from build123d import *

# Parameters (mm, degrees)
SKETCH1_R           = 1.5
BOSS_EXTRUDE1_DEPTH = 3
FILLET1_R           = 1


with BuildPart() as part:
    # Sketch1 → Boss-Extrude1 (new body)
    with BuildSketch(Plane.XY):
        with BuildLine():
            Line((-2.5, 0), (-2.5, -37.136851725))
            Line((-2.5, -37.136851725), (-7.28143986, -46.828388088))
            ThreePointArc((-7.28143986, -46.828388088), (-6.145564068, -50.176489966), (-2.79746219, -49.040614175))
            Line((-2.79746219, -49.040614175), (2.5, -38.303148275))
            Line((2.5, -38.303148275), (2.5, 0))
            ThreePointArc((2.5, 0), (0, 2.5), (-2.5, 0))
        make_face()
        Circle(SKETCH1_R, mode=Mode.SUBTRACT)
        with Locations((-5.039451025, -47.934501132)):
            Circle(SKETCH1_R, mode=Mode.SUBTRACT)
    extrude(amount=BOSS_EXTRUDE1_DEPTH)

    # Fillet1
    # the kernel refuses this fillet: 1 mm, written as the material it adds along each edge
    with BuildSketch(Plane(origin=(-2.5, -37.136851725, 0), x_dir=(0, 1, 0), z_dir=(0, 0, 1))) as fillet1_piece_1:
        with BuildLine():
            CenterArc((FILLET1_R * 0.23325930992, FILLET1_R), FILLET1_R, 243.74, 26.26)
            Line((-FILLET1_R * 0.209185907385, FILLET1_R * 0.103204466066), (0, 0))
            Line((0, 0), (FILLET1_R * 0.23325930992, 0))
        make_face()
    extrude(amount=3)
    # the kernel refuses this fillet: 1 mm, written as the material it takes off along each edge
    with BuildSketch(Plane(origin=(1.5, -38.069888965, 2), x_dir=(0.8967955339340403, -0.44244521730487674, 0), z_dir=(0, 0, 1))) as fillet1_2_piece_1_section:
        Polygon((0, 0), (FILLET1_R, 0), (FILLET1_R, FILLET1_R * 0.23325930992), (FILLET1_R * 0.896795533934, FILLET1_R * 0.442445217305), align=None)
    fillet1_2_piece_1 = extrude(amount=FILLET1_R, mode=Mode.PRIVATE)
    fillet1_2_piece_1 = fillet1_2_piece_1 - Plane(origin=(1.5, -38.069888965, 2), x_dir=(-0.9738571594268947, 0.22716124896861223, 0), z_dir=(0, 0, 1)) * Sphere(FILLET1_R, mode=Mode.PRIVATE)
    add(fillet1_2_piece_1, mode=Mode.SUBTRACT)
    with BuildSketch(Plane(origin=(1.5, -38.069888965, 1), x_dir=(0.8967955339340403, -0.44244521730487674, 0), z_dir=(0, 0, -1))) as fillet1_2_piece_2_section:
        Polygon((0, 0), (FILLET1_R, 0), (FILLET1_R, -FILLET1_R * 0.23325930992), (FILLET1_R * 0.896795533934, -FILLET1_R * 0.442445217305), align=None)
    fillet1_2_piece_2 = extrude(amount=FILLET1_R, mode=Mode.PRIVATE)
    fillet1_2_piece_2 = fillet1_2_piece_2 - Plane(origin=(1.5, -38.069888965, 1), x_dir=(-0.9738571594268947, 0.22716124896861223, 0), z_dir=(0, 0, -1)) * Sphere(FILLET1_R, mode=Mode.PRIVATE)
    add(fillet1_2_piece_2, mode=Mode.SUBTRACT)
    with BuildSketch(Plane(origin=(0, 0, 3), x_dir=(1, 0, 0), z_dir=(0, -1, 0))) as fillet1_2_piece_3:
        with BuildLine():
            CenterArc((2.5 - FILLET1_R, -FILLET1_R), FILLET1_R, 0, 90)
            Line((2.5, -FILLET1_R), (2.5, 0))
            Line((2.5, 0), (2.5 - FILLET1_R, 0))
        make_face()
    revolve(axis=Axis((0, 0, 3), (0, 0, 1)), revolution_arc=180, mode=Mode.SUBTRACT)
    with BuildSketch(Plane(origin=(0, 0, 0), x_dir=(1, 0, 0), z_dir=(0, -1, 0))) as fillet1_2_piece_4:
        with BuildLine():
            CenterArc((2.5 - FILLET1_R, FILLET1_R), FILLET1_R, 270, 90)
            Line((2.5, FILLET1_R), (2.5, 0))
            Line((2.5, 0), (2.5 - FILLET1_R, 0))
        make_face()
    revolve(axis=Axis((0, 0, 0), (0, 0, 1)), revolution_arc=180, mode=Mode.SUBTRACT)
    with BuildSketch(Plane(origin=(-2.5, 0, 3), x_dir=(0, 0, -1), z_dir=(0, -1, 0))) as fillet1_2_piece_5:
        with BuildLine():
            CenterArc((FILLET1_R, FILLET1_R), FILLET1_R, 180, 90)
            Line((0, FILLET1_R), (0, 0))
            Line((0, 0), (FILLET1_R, 0))
        make_face()
    extrude(amount=36.903592415, mode=Mode.SUBTRACT)
    with BuildSketch(Plane(origin=(-2.5, 0, 0), x_dir=(0, 0, 1), z_dir=(0, -1, 0))) as fillet1_2_piece_6:
        with BuildLine():
            CenterArc((FILLET1_R, -FILLET1_R), FILLET1_R, 90, 90)
            Line((0, -FILLET1_R), (0, 0))
            Line((0, 0), (FILLET1_R, 0))
        make_face()
    extrude(amount=36.903592415, mode=Mode.SUBTRACT)
    with BuildSketch(Plane(origin=(-2.603204466, -37.346037633, 3), x_dir=(0.8967955339340403, -0.4424452173048767, 0), z_dir=(-0.4424452173048767, -0.8967955339340403, 0))) as fillet1_2_piece_7:
        with BuildLine():
            CenterArc((FILLET1_R, -FILLET1_R), FILLET1_R, 90, 90)
            Line((0, -FILLET1_R), (0, 0))
            Line((0, 0), (FILLET1_R, 0))
        make_face()
    extrude(amount=10.573592415, mode=Mode.SUBTRACT)
    with BuildSketch(Plane(origin=(-2.603204466, -37.346037633, 0), x_dir=(0.8967955339340403, -0.4424452173048767, 0), z_dir=(-0.4424452173048767, -0.8967955339340403, 0))) as fillet1_2_piece_8:
        with BuildLine():
            CenterArc((FILLET1_R, FILLET1_R), FILLET1_R, 180, 90)
            Line((0, FILLET1_R), (0, 0))
            Line((0, 0), (FILLET1_R, 0))
        make_face()
    extrude(amount=10.573592415, mode=Mode.SUBTRACT)
    with BuildSketch(Plane(origin=(-5.039451025, -47.934501132, 3), x_dir=(-0.8967955339340404, 0.44244521730487624, 0), z_dir=(0.44244521730487624, 0.8967955339340404, 0))) as fillet1_2_piece_9:
        with BuildLine():
            CenterArc((2.5 - FILLET1_R, -FILLET1_R), FILLET1_R, 0, 90)
            Line((2.5, -FILLET1_R), (2.5, 0))
            Line((2.5, 0), (2.5 - FILLET1_R, 0))
        make_face()
    revolve(axis=Axis((-5.039451025, -47.934501132, 3), (0, 0, 1)), revolution_arc=180, mode=Mode.SUBTRACT)
    with BuildSketch(Plane(origin=(-5.039451025, -47.934501132, 0), x_dir=(-0.8967955339340404, 0.44244521730487624, 0), z_dir=(0.44244521730487624, 0.8967955339340404, 0))) as fillet1_2_piece_10:
        with BuildLine():
            CenterArc((2.5 - FILLET1_R, FILLET1_R), FILLET1_R, 270, 90)
            Line((2.5, FILLET1_R), (2.5, 0))
            Line((2.5, 0), (2.5 - FILLET1_R, 0))
        make_face()
    revolve(axis=Axis((-5.039451025, -47.934501132, 0), (0, 0, 1)), revolution_arc=180, mode=Mode.SUBTRACT)
    with BuildSketch(Plane(origin=(-2.79746219, -49.040614175, 3), x_dir=(-0.8967955339340403, 0.44244521730487674, 0), z_dir=(0.44244521730487674, 0.8967955339340403, 0))) as fillet1_2_piece_11:
        with BuildLine():
            CenterArc((FILLET1_R, -FILLET1_R), FILLET1_R, 90, 90)
            Line((0, -FILLET1_R), (0, 0))
            Line((0, 0), (FILLET1_R, 0))
        make_face()
    extrude(amount=11.739888965, mode=Mode.SUBTRACT)
    with BuildSketch(Plane(origin=(-2.79746219, -49.040614175, 0), x_dir=(-0.8967955339340403, 0.44244521730487674, 0), z_dir=(0.44244521730487674, 0.8967955339340403, 0))) as fillet1_2_piece_12:
        with BuildLine():
            CenterArc((FILLET1_R, FILLET1_R), FILLET1_R, 180, 90)
            Line((0, FILLET1_R), (0, 0))
            Line((0, 0), (FILLET1_R, 0))
        make_face()
    extrude(amount=11.739888965, mode=Mode.SUBTRACT)
    with BuildSketch(Plane(origin=(2.5, -38.303148275, 1), x_dir=(-0.4424452173048793, -0.896795533934039, 0), z_dir=(0, 0, 1))) as fillet1_2_piece_13:
        with BuildLine():
            CenterArc((FILLET1_R * 0.23325930992, -FILLET1_R), FILLET1_R, 90, 26.26)
            Line((-FILLET1_R * 0.209185907385, -FILLET1_R * 0.103204466066), (0, 0))
            Line((0, 0), (FILLET1_R * 0.23325930992, 0))
        make_face()
    extrude(amount=1, mode=Mode.SUBTRACT)
    with BuildSketch(Plane(origin=(2.5, -38.069888965, 3), x_dir=(-1, 0, 0), z_dir=(0, 1, 0))) as fillet1_2_piece_14:
        with BuildLine():
            CenterArc((FILLET1_R, -FILLET1_R), FILLET1_R, 90, 90)
            Line((0, -FILLET1_R), (0, 0))
            Line((0, 0), (FILLET1_R, 0))
        make_face()
    extrude(amount=38.069888965, mode=Mode.SUBTRACT)
    with BuildSketch(Plane(origin=(2.5, -38.069888965, 0), x_dir=(-1, 0, 0), z_dir=(0, 1, 0))) as fillet1_2_piece_15:
        with BuildLine():
            CenterArc((FILLET1_R, FILLET1_R), FILLET1_R, 180, 90)
            Line((0, FILLET1_R), (0, 0))
            Line((0, 0), (FILLET1_R, 0))
        make_face()
    extrude(amount=38.069888965, mode=Mode.SUBTRACT)
    with BuildSketch(Plane(origin=(0, 0, 0), x_dir=(1, 0, 0), z_dir=(0, -1, 0))) as fillet1_2_piece_16:
        with BuildLine():
            CenterArc((1.5 + FILLET1_R, FILLET1_R), FILLET1_R, 180, 90)
            Line((1.5, FILLET1_R), (1.5, 0))
            Line((1.5, 0), (1.5 + FILLET1_R, 0))
        make_face()
    revolve(axis=Axis((0, 0, 0), (0, 0, 1)), mode=Mode.SUBTRACT)
    with BuildSketch(Plane(origin=(0, 0, 3), x_dir=(1, 0, 0), z_dir=(0, -1, 0))) as fillet1_2_piece_17:
        with BuildLine():
            CenterArc((1.5 + FILLET1_R, -FILLET1_R), FILLET1_R, 90, 90)
            Line((1.5, -FILLET1_R), (1.5, 0))
            Line((1.5, 0), (1.5 + FILLET1_R, 0))
        make_face()
    revolve(axis=Axis((0, 0, 3), (0, 0, 1)), mode=Mode.SUBTRACT)
    with BuildSketch(Plane(origin=(-5.039451025, -47.934501132, 0), x_dir=(1, 0, 0), z_dir=(0, -1, 0))) as fillet1_2_piece_18:
        with BuildLine():
            CenterArc((1.5 + FILLET1_R, FILLET1_R), FILLET1_R, 180, 90)
            Line((1.5, FILLET1_R), (1.5, 0))
            Line((1.5, 0), (1.5 + FILLET1_R, 0))
        make_face()
    revolve(axis=Axis((-5.039451025, -47.934501132, 0), (0, 0, 1)), mode=Mode.SUBTRACT)
    with BuildSketch(Plane(origin=(-5.039451025, -47.934501132, 3), x_dir=(1, 0, 0), z_dir=(0, -1, 0))) as fillet1_2_piece_19:
        with BuildLine():
            CenterArc((1.5 + FILLET1_R, -FILLET1_R), FILLET1_R, 90, 90)
            Line((1.5, -FILLET1_R), (1.5, 0))
            Line((1.5, 0), (1.5 + FILLET1_R, 0))
        make_face()
    revolve(axis=Axis((-5.039451025, -47.934501132, 3), (0, 0, 1)), mode=Mode.SUBTRACT)
    with BuildSketch(Plane(origin=(-3.5, -36.903592415, 0), x_dir=(1, 0, 0), z_dir=(0, 1, 0))) as fillet1_2_piece_20:
        with BuildLine():
            CenterArc((1 + FILLET1_R, -FILLET1_R), FILLET1_R, 90, 90)
            Line((1, -FILLET1_R), (1, 0))
            Line((1, 0), (1 + FILLET1_R, 0))
        make_face()
    revolve(axis=Axis((-3.5, -36.903592415, 0), (0, 0, -1)), revolution_arc=26.26, mode=Mode.SUBTRACT)
    with BuildSketch(Plane(origin=(-3.5, -36.903592415, 3), x_dir=(1, 0, 0), z_dir=(0, 1, 0))) as fillet1_2_piece_21:
        with BuildLine():
            CenterArc((1 + FILLET1_R, FILLET1_R), FILLET1_R, 180, 90)
            Line((1 + FILLET1_R, 0), (1, 0))
            Line((1, 0), (1, FILLET1_R))
        make_face()
    revolve(axis=Axis((-3.5, -36.903592415, 3), (0, 0, -1)), revolution_arc=26.26, mode=Mode.SUBTRACT)


solid = part.part
For this review, take the finished solid that the model builds, in its own axes (mm). A direction names the side the tool comes from. Coordinates: 2 decimals unless noted, no trailing zeros. Loops run counter-clockwise (first coordinate to the right, second up) from the corner with the lowest first, then second, coordinate; pieces in that order, holes last. Notation, with made-up numbers: (49, 26.25) -> (79, 26.25) arc R25 ccw to (79, 40.25) -> close; hole circle Ø5 at (48, 56). An arc over 180 degrees is marked (long way). Write each question's results on one line, items separated by ' | '.
Q1. To check wall thickness, follow line 1 along X through (y, z) = (-15, 0.85); line 2 along Z through (x, y) = (2, -21.5); line 3 along Y through (x, z) = (-4, 2). State the ranges of each line that lie inside material, in increasing order. Write a range as [from, to].
Taken from the geometry:
line 1: [-2.49, 2.49] | line 2: [0.13, 2.87] | line 3: [-50.21, -49.02], [-46.85, -40.18]
Q2. Add section A-A, the plane y = -31.5. State the section outline as (x, z) points.
Taken from the geometry:
outline: (-2.5, 1) arc R1 ccw to (-1.5, 0) -> (1.5, 0) arc R1 ccw to (2.5, 1) -> (2.5, 2) arc R1 ccw to (1.5, 3) -> (-1.5, 3) arc R1 ccw to (-2.5, 2) -> close
Q3. Machinability: for faces 1 (the cylindrical face through (-2.199, -18.193, 2.715)), 2 (the cylindrical face through (-2.215, -18.193, 0.301)), 3 (the flat face through (-2.5, -18.2, 1.5)), 4 (the cylindrical face through (-0.49, -43.72, 0.3)), which of the approach directions +Z, -Z, +X, -X, +Y, -Y give a long, thin tool a straight path to every point of the face, cutting with its end or side? Answer none if there is none.
Taken from the geometry:
face 1: +Z, -X, +Y | face 2: -Z, -X, +Y | face 3: +Z, -Z, -X, +Y | face 4: -Z, +X, -Y
Q4. For pin 1 Ø4 at (x, y) = (0, 0) entering from -Z; pin 2 Ø3.5 at (x, y) = (-5.04, -47.93) entering from +Z; pin 3 Ø1.1 at (y, z) = (-10.5, 1.5) entering from -X, all flat-tipped, find the tip position at first contact; note any pin that passes through.
Taken from the geometry:
pin 1: z = 0.13 | pin 2: z = 2.67 | pin 3: x = -2.5
